Verification items for this drawing (mm, ordinates from the low corner). Round coordinates to 2 decimals unless told otherwise and drop trailing zeros. Loops run counter-clockwise (first coordinate to the right, second up) from the corner with the lowest first, then second, coordinate; pieces in that order, holes last. Notation, with made-up numbers: (35, -32) -> (75, -32) arc R33 ccw to (75, 4) -> close; hole circle Ø6 at (73, 60). An arc over 180 degrees is marked (long way). Use a Markdown table: item, result. Add a question column.
Q1. Release check for a two-part mould opening along Y. For the marked faces 1 and 2 record: released by +Y, released by -Y, zero draft, split by the parting line, or undercut.
Q2. Gauge pin test, flat end, axial feed: P1, Ø2.5, axis at x = 6.35, z = 3.175, coming from the +Y side. Record the tip position at first contact, or that the pin passes through.
Q3. Sectioned sample at A-A, the plane x = 57.15. Enter the section's corners in (y, z) (3 decimals), then the cut area to 3 significant figures.
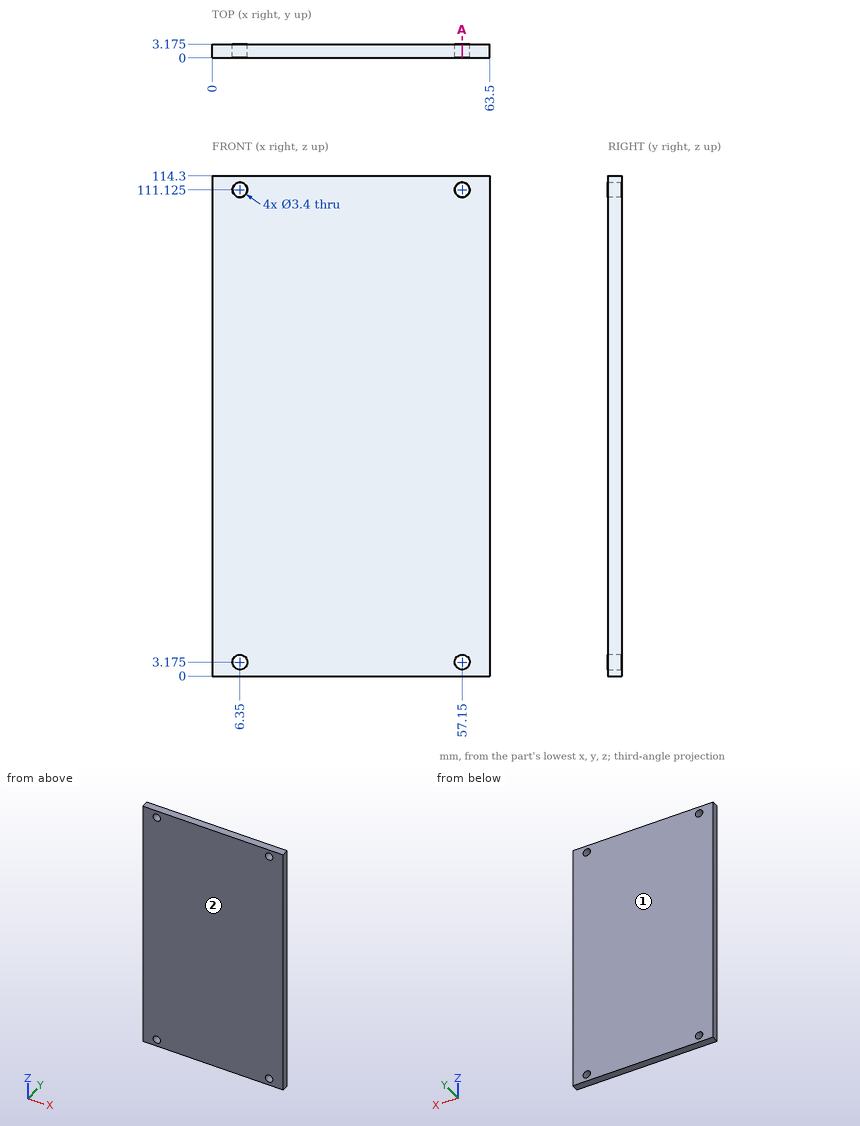
Values:
| question | item | result |
|---|---|---|
| 1 | face 1 | released by +Y |
| 1 | face 2 | released by -Y |
| 2 | P1 | through |
| 3 | outline | (0, 0) -> (3.175, 0) -> (3.175, 1.475) -> (0, 1.475) -> close; (0, 4.875) -> (3.175, 4.875) -> (3.175, 109.425) -> (0, 109.425) -> close; (0, 112.825) -> (3.175, 112.825) -> (3.175, 114.3) -> (0, 114.3) -> close |
| 3 | area | 341 mm^2 |
